Solid Edge part; units mm, degrees
sketch "Sketch1" plane through (0, 0, 0) normal (0, 0, 1) x (1, 0, 0)
  circle A0 centre (0, 0) radius 4.25
extrude "Protrusion1" add sketch "Sketch1" along normal blind 5
sketch "Sketch2" plane through (0, 0, 5) normal (0, 0, 1) x (1, 0, 0)
  circle A0 centre (0, 0) radius 2.5
extrude "ExtrudedProtrusion_2" add sketch "Sketch2" along normal blind 40
sketch "Sketch3" plane through (0, 0, 0) normal (0, 0, -1) x (-1, 0, 0)
  line L0 (2.25, 0) -> (1.125, 1.9486)
  line L1 (1.125, 1.9486) -> (-1.125, 1.9486)
  line L2 (-1.125, 1.9486) -> (-2.25, 0)
  line L3 (-2.25, 0) -> (-1.125, -1.9486)
  line L4 (-1.125, -1.9486) -> (1.125, -1.9486)
  line L5 (1.125, -1.9486) -> (2.25, 0)
extrude "ExtrudedCutout_1" cut sketch "Sketch3" against normal blind 2.6
properties material "Stainless steel"
Check sheet for the modelled part. Datum: model origin and axes. Units: mm. A direction names the side the tool comes from. Give positions to 0.01 mm unless a question says otherwise; leave off trailing zeros. Order: outer loops, then holes, each group sorted by start corner. A loop starts at its lowest first (then second) coordinate and runs counter-clockwise, first axis right, second up. Notation, with made-up numbers: M 65.5,61 L 82.5,61 A20 ccw 82.5,81 Z; hole C 17,65.5 d3. An arc over 180 degrees is marked long. Answer in a Markdown table with one row per item. Add a question column.
Q1. Release check for a two-part mould opening along Y. For faces 1 (the flat face through (-1.68, -0.99, 1.28)), 2 (the flat face through (0, 0, 45)), 3 (the cylindrical face through (2.285, -3.584, 2.465)) record: released by +Y, released by -Y, zero draft, split by the parting line, or undercut.
Q2. Sectioned sample at A-A, the plane x = 0. Record the boundary of the cut face in (y, z).
Q3. Gauge pin test, flat ends, axial feed: pin 1 Ø1.5 at (x, z) = (-3, 16) entering from +Y; pin 2 Ø0.7 at (x, z) = (-0.5, 0.5) entering from +Y; pin 3 Ø1.9 at (x, y) = (1, 0) entering from -Z. Record the tip position at first contact, or that the pin passes through.
Q4. Sectioned sample at C-C, the plane y = -1. Record the boundary of the cut face in (x, z), and give its area (3 significant figures).
Q5. Sectioned sample at D-D, the plane y = -3.25. Record the boundary of the cut face in (x, z), and give its area (3 significant figures).
Q6. Sectioned sample at B-B, the plane z = 42. Record the boundary of the cut face in (x, y), and give its area (3 significant figures).
Q7. Access from +Z, -Z, +X, -X, +Y, -Y to the whole of each face (thin tool, end or side, straight path). Record for faces 4 (the flat face through (1.695, -0.961, 1.282)), 5 (the cylindrical face through (-0.54, 2.44, 24.72)), 6 (the flat face through (2, -1, 0)).
Q8. Thickness scan on L1, parallel to Z at x = 2, y = 0.25; L2, parallel to Z at x = -1.5, y = 3.75; L3, parallel to Y at x = 0, z = 39.5. Record the ranges inside material, lowest first.
Verdict:
| question | item | result |
|---|---|---|
| 1 | face 1 | undercut |
| 1 | face 2 | zero draft |
| 1 | face 3 | split by the parting line |
| 2 | outline | M -4.25,0 L -1.95,0 L -1.95,2.6 L 1.95,2.6 L 1.95,0 L 4.25,0 L 4.25,5 L 2.5,5 L 2.5,45 L -2.5,45 L -2.5,5 L -4.25,5 Z |
| 3 | pin 1 | y = 1.09 |
| 3 | pin 2 | y = 4.25 |
| 3 | pin 3 | z = 2.6 |
| 4 | outline | M -4.13,0 L -1.67,0 L -1.67,2.6 L 1.67,2.6 L 1.67,0 L 4.13,0 L 4.13,5 L 2.29,5 L 2.29,45 L -2.29,45 L -2.29,5 L -4.13,5 Z |
| 4 | area | 216 mm² |
| 5 | outline | M -2.74,0 L 2.74,0 L 2.74,5 L -2.74,5 Z |
| 5 | area | 27.4 mm² |
| 6 | outline | C 0,0 d5 |
| 6 | area | 19.6 mm² |
| 7 | face 4 | -Z |
| 7 | face 5 | +Z |
| 7 | face 6 | -Z, +X, -X, +Y, -Y |
| 8 | L1 | 2.6 to 45 |
| 8 | L2 | 0 to 5 |
| 8 | L3 | -2.5 to 2.5 |
